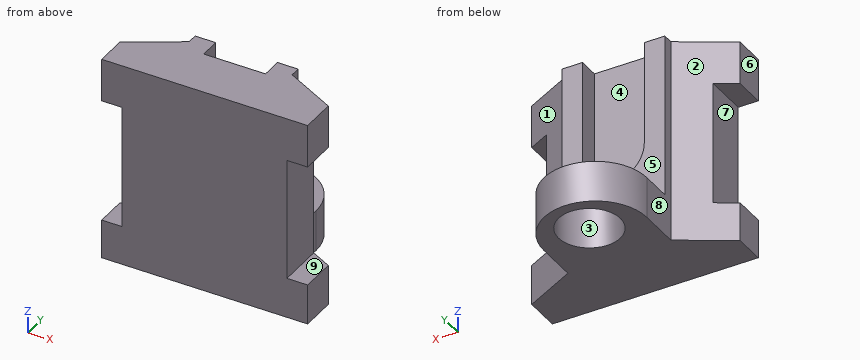
```python
from build123d import *

# Parameters (mm, degrees)
SKETCH1_W               = 100
SKETCH1_H               = 30
BOSS_EXTRUDE1_DEPTH     = 100
SKETCH2_W               = 50
SKETCH2_H               = 5
BOSS_EXTRUDE2_DEPTH     = 100
BOSS_EXTRUDE3_DEPTH     = 20
SKETCH4_R               = 15
CUT_EXTRUDE2_DEPTH      = 20
SKETCH5_W               = 9.754337327
SKETCH5_H               = 60.08086333
CUT_EXTRUDE3_DEPTH      = 55.43877551
CUT_EXTRUDE3_DEPTH_BACK = 21.56122449
SKETCH6_W               = 10.053487374
SKETCH6_H               = 59.424714791
CUT_EXTRUDE4_DEPTH      = 46
CUT_EXTRUDE4_DEPTH_BACK = 31
CUT_EXTRUDE5_DEPTH      = 10
CUT_EXTRUDE9_DEPTH      = 130
CUT_EXTRUDE11_DEPTH     = 130


with BuildPart() as part:
    # Sketch1 → Boss-Extrude1 (new body)
    with BuildSketch(Plane.XY):
        with Locations((13.775510204, -5.56122449)):
            Rectangle(SKETCH1_W, SKETCH1_H)
    extrude(amount=BOSS_EXTRUDE1_DEPTH)

    # Sketch2 → Boss-Extrude2 (add)
    with BuildSketch(Plane.XY):
        with Locations((13.775510204, 11.93877551)):
            Rectangle(SKETCH2_W, SKETCH2_H)
    extrude(amount=BOSS_EXTRUDE2_DEPTH)

    # Sketch3 → Boss-Extrude3 (add)
    with BuildSketch(Plane.XY):
        with BuildLine():
            Line((-11.224489796, 14.43877551), (38.775510204, 14.43877551))
            Line((38.775510204, 14.43877551), (38.775510204, 29.43877551))
            ThreePointArc((38.775510204, 29.43877551), (13.775510204, 54.43877551), (-11.224489796, 29.43877551))
            Line((-11.224489796, 29.43877551), (-11.224489796, 14.43877551))
        make_face()
    extrude(amount=BOSS_EXTRUDE3_DEPTH)

    # Sketch4 → Cut-Extrude2 (cut)
    with BuildSketch(Plane.XY.offset(20)):
        with Locations((13.775510204, 34.43877551)):
            Circle(SKETCH4_R)
    extrude(amount=-CUT_EXTRUDE2_DEPTH, mode=Mode.SUBTRACT)

    # Sketch5 → Cut-Extrude3 (cut, two sides)
    with BuildSketch(Plane(origin=(0, 0, 0), x_dir=(1, 0, 0), z_dir=(0, 1, 0))) as cut_extrude3_sk:
        with Locations((-31.347321132, -49.035804096)):
            Rectangle(SKETCH5_W, SKETCH5_H)
    extrude(amount=CUT_EXTRUDE3_DEPTH, mode=Mode.SUBTRACT)
    extrude(cut_extrude3_sk.sketch, amount=-CUT_EXTRUDE3_DEPTH_BACK, mode=Mode.SUBTRACT)

    # Sketch6 → Cut-Extrude4 (cut, two sides)
    with BuildSketch(Plane(origin=(0, 9.43877551, 0), x_dir=(1, 0, 0), z_dir=(0, 1, 0))) as cut_extrude4_sk:
        with Locations((58.748766517, -49.363878365)):
            Rectangle(SKETCH6_W, SKETCH6_H)
    extrude(amount=CUT_EXTRUDE4_DEPTH, mode=Mode.SUBTRACT)
    extrude(cut_extrude4_sk.sketch, amount=-CUT_EXTRUDE4_DEPTH_BACK, mode=Mode.SUBTRACT)

    # Sketch7 → Cut-Extrude5 (cut)
    with BuildSketch(Plane(origin=(0, 14.43877551, 0), x_dir=(1, 0, 0), z_dir=(0, 1, 0))):
        with BuildLine():
            Line((-1.224489796, -90), (-1.224489796, -100))
            Line((-1.224489796, -100), (28.775510204, -100))
            Line((28.775510204, -100), (28.775510204, -90))
            Line((28.775510204, -90), (28.775510204, -49.395873988))
            ThreePointArc((28.775510204, -49.395873988), (13.775510204, -34.395873988), (-1.224489796, -49.395873988))
            Line((-1.224489796, -49.395873988), (-1.224489796, -90))
        make_face()
    extrude(amount=-CUT_EXTRUDE5_DEPTH, mode=Mode.SUBTRACT)

    # Sketch8 → Cut-Extrude9 (cut)
    with BuildSketch(Plane.XY.offset(100)):
        Polygon((63.775510204, 3.25154294), (63.775510204, 9.43877551), (51.275510204, 9.43877551), align=None)
        Polygon((-36.224489796, 9.43877551), (-23.724489796, 9.43877551), (-36.224489796, 3.25154294), align=None)
    extrude(amount=-CUT_EXTRUDE9_DEPTH, mode=Mode.SUBTRACT)

    # Sketch9 → Cut-Extrude11 (cut)
    with BuildSketch(Plane.XY.offset(100)):
        Polygon((-11.224489796, 9.43877551), (-36.224489796, -5.508285905), (-36.224489796, 9.273925271), (-21.818059328, 14.371872445), align=None)
        Polygon((38.775510204, 9.43877551), (67.925947804, 9.43877551), (67.925947804, -5.508285905), align=None)
    extrude(amount=-CUT_EXTRUDE11_DEPTH, mode=Mode.SUBTRACT)


solid = part.part
```
Work out the finished part from the listing and answer in its coordinate system (mm). Face numbers are marked on the shaded views. A direction names the side the tool comes from. Coordinates: 2 decimals unless noted, no trailing zeros. Order: outer loops, then holes, each group sorted by start corner. A loop starts at its lowest first (then second) coordinate and runs counter-clockwise, first axis right, second up. Notation, with made-up numbers: (-22.5, -25) - (-13.5, -25) arc R32 cw to (-13.5, 6) - close; hole circle Ø7 at (6, 54). An arc over 180 degrees is marked (long way). Answer as a JSON object with one key per item and string values.
1. Consider line 1 (Y direction, x = 10.5, z = 27.5); line 2 (Y direction, x = 5.5, z = 47.5); line 3 (X direction, y = 34.5, z = 7). Determine where each line is inside the solid, lowest interval first.
Output values:
{"line 1": "y = -20.56 to 14.44", "line 2": "y = -20.56 to 4.44", "line 3": "x = -10.71 to -1.22, 28.78 to 38.26"}
2. Each of these flat-tipped pins is pushed along its axis until it touches: P1, Ø24, axis at x = 13.78, y = 34.44, coming from the -Z side; P2, Ø8, axis at y = 7.5, z = 65.5, coming from the -X side; P3, Ø1, axis at x = 48.5, z = 63.5, coming from the +Y side; P4, Ø2, axis at y = 0, z = 39.5, coming from the -X side. Where does it stop, or does it pass through?
Output values:
{"P1": "passes through", "P2": "stops at x = -21.16", "P3": "stops at y = 4.71", "P4": "stops at x = -26.47"}
3. Find section D-D on y = -14. Determine the outline of the cut face in (x, z).
Output values:
{"outline": "(-36.22, 0) - (63.78, 0) - (63.78, 19.65) - (53.72, 19.65) - (53.72, 79.08) - (63.78, 79.08) - (63.78, 100) - (-36.22, 100) - (-36.22, 79.08) - (-26.47, 79.08) - (-26.47, 19) - (-36.22, 19) - close"}
4. Find section A-A on y = 36.5. Determine the outline of the cut face in (x, z), plus the area to 3 significant figures.
Output values:
{"outline": "(-10.21, 0) - (-1.08, 0) - (-1.08, 20) - (-10.21, 20) - close; (28.63, 0) - (37.76, 0) - (37.76, 20) - (28.63, 20) - close", "area": "365 mm²"}
5. A tool of negligible diameter and unlimited length cuts with its end or side. For the marked faces 5, 6, 7, 8 and 9, from which of +Z, -Z, +X, -X, +Y, -Y can it reach the whole face along a straight path? Write none if from no direction.
Output values:
{"face 5": "+Z, +X, -X, +Y", "face 6": "+Z, -Z, -X, +Y, -Y", "face 7": "-X, +Y, -Y", "face 8": "+Z, -Z, -X, +Y", "face 9": "+X, +Y, -Y"}
6. Find section B-B on x = 3.5. Determine the outline of the cut face in (y, z), plus the area to 3 significant figures.
Output values:
{"outline": "(-20.56, 0) - (23.51, 0) - (23.51, 20) - (14.44, 20) - (14.44, 38.47) - (4.44, 38.47) - (4.44, 100) - (-20.56, 100) - close; (45.37, 0) - (52.23, 0) - (52.23, 20) - (45.37, 20) - close", "area": "3,200 mm²"}
7. Find section C-C on z = 88.5. Determine the outline of the cut face in (x, y).
Output values:
{"outline": "(-36.22, -20.56) - (63.78, -20.56) - (63.78, -3.38) - (38.78, 9.44) - (38.78, 14.44) - (28.78, 14.44) - (28.78, 4.44) - (-1.22, 4.44) - (-1.22, 14.44) - (-11.22, 14.44) - (-11.22, 9.44) - (-36.22, -5.51) - close"}
8. The mould has two halves that part along X. Classify the marked faces 1, 2, 3 and 4: +X half, -X half, draft (parallel to the pull), parting line (faces both ways), or undercut.
Output values:
{"face 1": "+X half", "face 2": "-X half", "face 3": "undercut", "face 4": "undercut"}
